from build123d import *

# Parameters (mm, degrees)
BOSS_EXTRUDE1_DEPTH  = 28.9
FILLET1_R            = 2.54
M3_CLEARANCE_HOLE1_D = 3.4


with BuildPart() as part:
    # Sketch1 → Boss-Extrude1 (new body)
    with BuildSketch(Plane(origin=(0, 0, 0), x_dir=(1, 0, 0), z_dir=(0, 1, 0))):
        with BuildLine():
            Line((9.16515139, 4), (17.036725037, 4))
            ThreePointArc((17.036725037, 4), (0, 17.5), (-17.036725037, 4))
            Line((-17.036725037, 4), (-9.16515139, 4))
            ThreePointArc((-9.16515139, 4), (0, 10), (9.16515139, 4))
        make_face()
        with BuildLine():
            Line((9.16515139, -4), (17.036725037, -4))
            ThreePointArc((17.036725037, -4), (17.383795445, -2.013369296), (17.5, 0))
            ThreePointArc((17.5, 0), (17.383795445, 2.013369296), (17.036725037, 4))
            Line((17.036725037, 4), (9.16515139, 4))
            ThreePointArc((9.16515139, 4), (9.789063129, 2.043096437), (10, 0))
            ThreePointArc((10, 0), (9.789063129, -2.043096437), (9.16515139, -4))
        make_face()
        with BuildLine():
            ThreePointArc((-17.036725037, 4), (-17.5, 0), (-17.036725037, -4))
            Line((-17.036725037, -4), (-9.16515139, -4))
            ThreePointArc((-9.16515139, -4), (-10, 0), (-9.16515139, 4))
            Line((-9.16515139, 4), (-17.036725037, 4))
        make_face()
        with BuildLine():
            ThreePointArc((-17.036725037, -4), (0, -17.5), (17.036725037, -4))
            Line((17.036725037, -4), (9.16515139, -4))
            ThreePointArc((9.16515139, -4), (0, -10), (-9.16515139, -4))
            Line((-9.16515139, -4), (-17.036725037, -4))
        make_face()
        with BuildLine():
            Line((17.036725037, -4), (20, -4))
            Line((20, -4), (20, 4))
            Line((20, 4), (17.036725037, 4))
            ThreePointArc((17.036725037, 4), (17.383795445, 2.013369296), (17.5, 0))
            ThreePointArc((17.5, 0), (17.383795445, -2.013369296), (17.036725037, -4))
        make_face()
        with BuildLine():
            ThreePointArc((20, 4), (24, 0), (20, -4))
            Line((20, -4), (20, 4))
        make_face()
        with BuildLine():
            Line((-20, -4), (-20, 4))
            ThreePointArc((-20, 4), (-24, 0), (-20, -4))
        make_face()
        with BuildLine():
            Line((-20, -4), (-17.036725037, -4))
            ThreePointArc((-17.036725037, -4), (-17.5, 0), (-17.036725037, 4))
            Line((-17.036725037, 4), (-20, 4))
            Line((-20, 4), (-20, -4))
        make_face()
    extrude(amount=BOSS_EXTRUDE1_DEPTH)

    # Fillet1
    fillet1_edges = [part.edges().sort_by_distance(p)[0] for p in [
        (-17.036725037, 14.45, 4),
        (-17.036725037, 14.45, -4),
        (17.036725037, 14.45, -4),
        (17.036725037, 14.45, 4),
    ]]
    fillet(fillet1_edges, radius=FILLET1_R)

    # M3 Clearance Hole1 (through all)
    with Locations(Plane(origin=(0, 28.9, 0), x_dir=(1, 0, 0), z_dir=(0, 1, 0))):
        with Locations((-20, 0), (20, 0)):
            Hole(M3_CLEARANCE_HOLE1_D / 2)


solid = part.part
Geometry check sheet. Reference: the model listing, model coordinates, mm. A direction names the side the tool comes from. Round coordinates to 2 decimals unless told otherwise and drop trailing zeros. Loops run counter-clockwise (first coordinate to the right, second up) from the corner with the lowest first, then second, coordinate; pieces in that order, holes last.
Item 1: Thickness scan on line 1 (Z direction, x = 20, y = 6.5); line 2 (X direction, y = 27.5, z = 1); line 3 (Z direction, x = 9, y = 4). Record the ranges inside material, lowest first.
Item 2: Cross-section at B-B on z = -1. Record the boundary of the cut face in (x, y).
Item 3: Cross-section at A-A on y = 23.5. Record the boundary of the cut face in (x, z), then the cut area to 3 significant figures.
Item 4: Access from +Z, -Z, +X, -X, +Y, -Y to the whole of each face (thin tool, end or side, straight path). Record for faces 1 (the flat face through (19.5, 14.2, -4)), 2 (the flat face through (19.5, 14.2, 4)), 3 (the flat face through (-19.5, 14.2, 4)).
Item 5: Gauge pin test, flat ends, axial feed: pin 1 (0.8 mm diameter, centred on x = 19.5, y = 19, fed in from +Z); pin 2 (10 mm diameter, centred on x = 15, y = 10, fed in from -Z); pin 3 (2 mm diameter, centred on x = -20, z = 0, fed in from +Y); pin 4 (1.5 mm diameter, centred on x = -18, y = 5, fed in from -Z). Record the tip position at first contact, or that the pin passes through.
Item 6: Cross-section at C-C on x = 6. Record the boundary of the cut face in (y, z), then the cut area to 3 significant figures.
Item 7: Cross-section at D-D on z = 6.5. Record the boundary of the cut face in (x, y).
Item 8: Mould release check, pull along Z, two halves, no side actions. Record for faces 4 (the cylindrical face through (-17.487, 14.652, 4.459)), 5 (the cylindrical face through (18.43, 14.25, 0.65)), 6 (the cylindrical face through (0.303, 14.248, -17.497)): pulls with the +Z half, pulls with the -Z half, needs draft (parallel to the pull), parting line crosses it, or undercut.
Answer sheet:
1. line 1: z = -4 to -1.7, 1.7 to 4
1. line 2: x = -23.87 to -21.37, -18.63 to -9.95, 9.95 to 18.63, 21.37 to 23.87
1. line 3: z = -15.01 to -4.36, 4.36 to 15.01
2. outline: (-23.87, 0) - (-21.37, 0) - (-21.37, 28.9) - (-23.87, 28.9) - close; (-18.63, 0) - (-9.95, 0) - (-9.95, 28.9) - (-18.63, 28.9) - close; (9.95, 0) - (18.63, 0) - (18.63, 28.9) - (9.95, 28.9) - close; (21.37, 0) - (23.87, 0) - (23.87, 28.9) - (21.37, 28.9) - close
3. outline: (-20, -4) - (-18.94, -4) arc R2.54 cw to (-16.54, -5.71) arc R17.5 ccw to (16.54, -5.71) arc R2.54 cw to (18.94, -4) - (20, -4) arc R4 ccw to (20, 4) - (18.94, 4) arc R2.54 cw to (16.54, 5.71) arc R17.5 ccw to (-16.54, 5.71) arc R2.54 cw to (-18.94, 4) - (-20, 4) arc R4 ccw to start; hole circle Ø3.4 at (-20, 0); hole circle Ø20 at (0, 0); hole circle Ø3.4 at (20, 0)
3. area: 725 mm2
4. face 1: -Z, +X, +Y, -Y
4. face 2: +Z, +X, +Y, -Y
4. face 3: +Z, -X, +Y, -Y
5. pin 1: stops at z = 4
5. pin 2: stops at z = -14.36
5. pin 3: passes through
5. pin 4: stops at z = -4.65
6. outline: (0, -16.44) - (28.9, -16.44) - (28.9, -8) - (0, -8) - close; (0, 8) - (28.9, 8) - (28.9, 16.44) - (0, 16.44) - close
6. area: 488 mm2
7. outline: (-16.25, 0) - (-7.6, 0) - (-7.6, 28.9) - (-16.25, 28.9) - close; (7.6, 0) - (16.25, 0) - (16.25, 28.9) - (7.6, 28.9) - close
8. face 4: pulls with the +Z half
8. face 5: undercut
8. face 6: pulls with the -Z half
